For this review, take the finished solid that the model builds, in its own axes (mm). Give positions to 0.01 mm unless a question says otherwise; leave off trailing zeros. Loops run counter-clockwise (first coordinate to the right, second up) from the corner with the lowest first, then second, coordinate; pieces in that order, holes last. Notation, with made-up numbers: M 48,42 L 91,42 A21 ccw 91,65 Z; hole C 35.25,47.25 d3. An arc over 180 degrees is marked long. Use CSV: the item, a comma, the result in double quotes. Start each with the question number.
1. Take a section at B-B, the plane y = 1. Write out the cut boundary in (x, z).
2. Take a section at A-A, the plane z = 10. Write out the cut boundary in (x, y).
3. Insertion check: P1, Ø8, axis at x = -32.5, z = 10, coming from the -Y side. The pin has a flat end and moves straight along its axis. Give the tip position at first contact, or say it passes through.
4. The part is to be moulded in two halves that separate along X. For faces 1 (the face through (-34, 0, 12)), 2 (the face through (31.96, -0.04, -7.56)), 3 (the face through (57.5, 0, 0)), 4 (the face through (-1, -2.5, 0)), say which applies: pulls with the +X half, pulls with the -X half, needs draft (parallel to the pull), parting line crosses it, or undercut.
5. To check wall thickness, follow line 1 (X direction, y = 1.2, z = 10); line 2 (Z direction, x = -32.5, y = 0.6); line 3 (X direction, y = 2.05, z = 9.5). State the ranges of each line that lie inside material, in increasing order. Write a range as [from, to].
from build123d import *

# Parameters (mm, degrees)
SKETCH2_W           = 115
SKETCH2_H           = 40
SKETCH2_R           = 2.5
BOSS_EXTRUDE1_DEPTH = 2.5


with BuildPart() as part:
    # Sketch2 → Boss-Extrude1 (new body, symmetric)
    with BuildSketch(Plane(origin=(0, 0, 0), x_dir=(1, 0, 0), z_dir=(0, 1, 0))):
        Rectangle(SKETCH2_W, SKETCH2_H)
        with Locations((-32.5, 10)):
            Circle(SKETCH2_R, mode=Mode.SUBTRACT)
        with Locations((32.5, 10)):
            Circle(SKETCH2_R, mode=Mode.SUBTRACT)
        with Locations((32.5, -10)):
            Circle(SKETCH2_R, mode=Mode.SUBTRACT)
        with Locations((-32.5, -10)):
            Circle(SKETCH2_R, mode=Mode.SUBTRACT)
    extrude(amount=BOSS_EXTRUDE1_DEPTH, both=True)


solid = part.part
Result set:
1,outline,"M -57.5,-20 L 57.5,-20 L 57.5,20 L -57.5,20 Z; hole C -32.5,-10 d5; hole C -32.5,10 d5; hole C 32.5,-10 d5; hole C 32.5,10 d5"
2,outline,"M -57.5,-2.5 L -35,-2.5 L -35,2.5 L -57.5,2.5 Z; M -30,-2.5 L 30,-2.5 L 30,2.5 L -30,2.5 Z; M 35,-2.5 L 57.5,-2.5 L 57.5,2.5 L 35,2.5 Z"
3,P1,"y = -2.5"
4,face 1,"undercut"
4,face 2,"undercut"
4,face 3,"pulls with the +X half"
4,face 4,"needs draft"
5,line 1,"[-57.5, -35], [-30, 30], [35, 57.5]"
5,line 2,"[-20, -12.5], [-7.5, 7.5], [12.5, 20]"
5,line 3,"[-57.5, -34.95], [-30.05, 30.05], [34.95, 57.5]"
